```python
from build123d import *

# Parameters (mm, degrees)
SKETCH_1_W             = 130
SKETCH_1_H             = 125
EXTRUDE_1_DEPTH        = 50
SKETCH_2_R             = 6
CUT_EXTRUDE_1_DEPTH    = 51
FILLET_1_R             = 2
SKETCH_4_R             = 11.5
CUT_EXTRUDE_2_DEPTH    = 2
MM_4_D                 = 11
MM_4_DEPTH             = 25
MM_4_TIP               = 3.304733405
MM_4_2_D               = 11
MM_4_2_DEPTH           = 25
MM_4_2_TIP             = 3.304733405
HOLE_WIZARD_M5_1_D     = 4.2
HOLE_WIZARD_M5_1_DEPTH = 12
HOLE_WIZARD_M5_1_TIP   = 1.2618073
MM_3_D                 = 4
MM_3_DEPTH             = 56
MM_3_TIP               = 1.201721238
MM_4_3_D               = 4
MM_4_3_DEPTH           = 87
MM_4_3_TIP             = 1.201721238
MM_5_D                 = 4
M10X1_0_1_D            = 9
M10X1_0_1_DEPTH        = 14
M10X1_0_1_TIP          = 2.703872786


with BuildPart() as part:
    # 草图1 → 凸台-拉伸1 (new body)
    with BuildSketch(Plane(origin=(0, 0, 0), x_dir=(1, 0, 0), z_dir=(0, 1, 0))):
        Rectangle(SKETCH_1_W, SKETCH_1_H)
    extrude(amount=EXTRUDE_1_DEPTH)

    # 草图2 → 切除-拉伸1 (cut, through all)
    with BuildSketch(Plane(origin=(0, 50, 0), x_dir=(1, 0, 0), z_dir=(0, 1, 0))):
        with Locations((-55, 52.5)):
            Circle(SKETCH_2_R)
        with Locations((55, 52.5)):
            Circle(SKETCH_2_R)
        with Locations((55, -52.5)):
            Circle(SKETCH_2_R)
        with Locations((-55, -52.5)):
            Circle(SKETCH_2_R)
    extrude(amount=-CUT_EXTRUDE_1_DEPTH, mode=Mode.SUBTRACT)

    # 圆角1
    fillet_1_edges = [part.edges().sort_by_distance(p)[0] for p in [
        (65, 25, 62.5),
        (-65, 25, 62.5),
        (-65, 25, -62.5),
        (65, 25, -62.5),
    ]]
    fillet(fillet_1_edges, radius=FILLET_1_R)

    # 草图4 → 切除-拉伸2 (cut)
    with BuildSketch(Plane.XZ):
        with Locations((-35, -27.5)):
            Circle(SKETCH_4_R)
        with Locations((5, 2.5)):
            Circle(SKETCH_4_R)
    extrude(amount=-CUT_EXTRUDE_2_DEPTH, mode=Mode.SUBTRACT)

    # mm _4
    with Locations(Plane(origin=(0, 2, 0), x_dir=(-1, 0, 0), z_dir=(0, -1, 0))):
        with Locations((-5, -2.5)):
            Hole(MM_4_D / 2, depth=MM_4_DEPTH)
            with Locations((0, 0, -(MM_4_DEPTH + MM_4_TIP / 2))):  # 118° drill point
                Cone(0, MM_4_D / 2, MM_4_TIP, mode=Mode.SUBTRACT)

    # mm _4 2
    with Locations(Plane(origin=(0, 2, 0), x_dir=(-1, 0, 0), z_dir=(0, -1, 0))):
        with Locations((35, 27.5)):
            Hole(MM_4_2_D / 2, depth=MM_4_2_DEPTH)
            with Locations((0, 0, -(MM_4_2_DEPTH + MM_4_2_TIP / 2))):  # 118° drill point
                Cone(0, MM_4_2_D / 2, MM_4_2_TIP, mode=Mode.SUBTRACT)

    # M5 螺纹孔1
    with Locations(Plane.XY.offset(62.5)):
        with Locations((-34.5, 45), (5.5, 45), (5.5, 5), (-34.5, 5)):
            Hole(HOLE_WIZARD_M5_1_D / 2, depth=HOLE_WIZARD_M5_1_DEPTH)
            with Locations((0, 0, -(HOLE_WIZARD_M5_1_DEPTH + HOLE_WIZARD_M5_1_TIP / 2))):  # 118° drill point
                Cone(0, HOLE_WIZARD_M5_1_D / 2, HOLE_WIZARD_M5_1_TIP, mode=Mode.SUBTRACT)

    # 大小mm 暗销孔3
    with Locations(Plane.XY.offset(62.5)):
        with Locations((3.5, 25)):
            Hole(MM_3_D / 2, depth=MM_3_DEPTH)
            with Locations((0, 0, -(MM_3_DEPTH + MM_3_TIP / 2))):  # 118° drill point
                Cone(0, MM_3_D / 2, MM_3_TIP, mode=Mode.SUBTRACT)

    # mm _4 3
    with Locations(Plane.XY.offset(62.5)):
        with Locations((-32.5, 25)):
            Hole(MM_4_3_D / 2, depth=MM_4_3_DEPTH)
            with Locations((0, 0, -(MM_4_3_DEPTH + MM_4_3_TIP / 2))):  # 118° drill point
                Cone(0, MM_4_3_D / 2, MM_4_3_TIP, mode=Mode.SUBTRACT)

    # 大小mm 暗销孔5 (through all)
    with Locations(Plane.XY.offset(62.5)):
        with Locations((-14.5, 43), (-14.5, 7)):
            Hole(MM_5_D / 2)

    # M10x1.0 螺纹孔1
    with Locations(Plane(origin=(0, 0, -62.5), x_dir=(-1, 0, 0), z_dir=(0, 0, -1))):
        with Locations((14.5, 43), (14.5, 7)):
            Hole(M10X1_0_1_D / 2, depth=M10X1_0_1_DEPTH)
            with Locations((0, 0, -(M10X1_0_1_DEPTH + M10X1_0_1_TIP / 2))):  # 118° drill point
                Cone(0, M10X1_0_1_D / 2, M10X1_0_1_TIP, mode=Mode.SUBTRACT)


solid = part.part
```
Could you check a few things on this model? Use its own coordinates, in mm. A direction names the side the tool comes from. Coordinates: 2 decimals unless noted, no trailing zeros. Order: outer loops, then holes, each group sorted by start corner. A loop starts at its lowest first (then second) coordinate and runs counter-clockwise, first axis right, second up. Notation, with made-up numbers: M 87,64 L 96,64 A23 ccw 96,100 Z; hole C 60.5,36.5 d5. An arc over 180 degrees is marked long. Use a Markdown table: item, result. Add a question column.
Q1. I want a section at D-D on y = 18.5. List the corners of the cut face in (x, z) for me, then the cut area to 3 significant figures.
Q2. I'm going to push flat-ended pins straight in: pin 1 (14.5 mm diameter, centred on x = -35, z = -27.5, fed in from -Y); pin 2 (2.5 mm diameter, centred on x = -34.5, y = 5, fed in from +Z). Where does each tip first touch, or does it pass through?
Q3. If I drill on L1, parallel to Y at x = -14, z = -55; L2, parallel to X at y = 23.5, z = 56.5; L3, parallel to Y at x = -13, z = -30, over which ranges is the centre line in solid material (lowest first)?
Q4. We'd pull the mould along Y, two halves only. Please class faces 1 (the cylindrical face through (-13.026, 8.352, 6.985)), 2 (the cylindrical face through (49.006, 25.35, 52.236)), 3 (the conical face through (5.76, 29.73, 3.08)): pulls with the +Y half, pulls with the -Y half, needs draft (parallel to the pull), parting line crosses it, or undercut.
Q5. I want a section at A-A on z = -52.5. List the corners of the cut face in (x, y) for me.
Q6. I want a section at B-B on x = -14.5. List the corners of the cut face in (y, z) for me.
Q7. Which directions (+Z, -Z, +X, -X, +Y, -Y) give clear straight access to the entire face, cutting with the end or side of a thin tool? Please do faces 4 (the flat face through (10, 2, 5.2)), 5 (the flat face through (65, 25, 1)), 6 (the cylindrical face through (-34.347, 24.234, 18.473)).
Q8. I want a section at C-C on y = 35. List the corners of the cut face in (x, z) for me.
Checked values:
| question | item | result |
|---|---|---|
| 1 | outline | M -65,-60.5 A2 ccw -63,-62.5 L 63,-62.5 A2 ccw 65,-60.5 L 65,60.5 A2 ccw 63,62.5 L -63,62.5 A2 ccw -65,60.5 Z; hole C -55,-52.5 d12; hole C -55,52.5 d12; hole C -35,-27.5 d11; hole C 5,2.5 d11; hole C 55,-52.5 d12; hole C 55,52.5 d12 |
| 1 | area | 15,600 mm² |
| 2 | pin 1 | y = 2 |
| 2 | pin 2 | z = 49.99 |
| 3 | L1 | 0 to 2.53, 11.47 to 38.53, 47.47 to 50 |
| 3 | L2 | -65 to -59.47, -50.53 to -33.82, -31.18 to 2.18, 4.82 to 50.53, 59.47 to 65 |
| 3 | L3 | 0 to 5.68, 8.32 to 41.68, 44.32 to 50 |
| 4 | face 1 | undercut |
| 4 | face 2 | needs draft |
| 4 | face 3 | pulls with the -Y half |
| 5 | outline | M -65,0 L -61,0 L -61,50 L -65,50 Z; M -49,0 L 49,0 L 49,50 L -49,50 Z; M 61,0 L 65,0 L 65,50 L 61,50 Z; hole C -14.5,7 d9; hole C -14.5,43 d9 |
| 6 | outline | M 0,-62.5 L 2.5,-62.5 L 2.5,-48.5 L 5,-47 L 5,62.5 L 0,62.5 Z; M 9,-47 L 11.5,-48.5 L 11.5,-62.5 L 38.5,-62.5 L 38.5,-48.5 L 41,-47 L 41,62.5 L 9,62.5 Z; M 45,-47 L 47.5,-48.5 L 47.5,-62.5 L 50,-62.5 L 50,62.5 L 45,62.5 Z |
| 7 | face 4 | -Y |
| 7 | face 5 | +Z, -Z, +X, +Y, -Y |
| 7 | face 6 | +Z |
| 8 | outline | M -65,-60.5 A2 ccw -63,-62.5 L 63,-62.5 A2 ccw 65,-60.5 L 65,60.5 A2 ccw 63,62.5 L -63,62.5 A2 ccw -65,60.5 Z; hole C -55,-52.5 d12; hole C -55,52.5 d12; hole C 55,-52.5 d12; hole C 55,52.5 d12 |
